from build123d import *

# Parameters (mm, degrees)
F0_W         = 125
F0_H         = 35
F1_DEPTH     = 50
F2_T         = -2.5
F3_T1_DEPTH  = 150
F5_DEPTH     = 47
F6_W         = 123.983182013
F6_H         = 1.5
F7_DEPTH     = 60
F8_T4_DEPTH  = 136.8415969529
F8_T9_DEPTH  = 123.983182013
F8_T14_DEPTH = 136.8415969529


# Not quite as in the source:
# - a fillet or chamfer that OpenCascade refuses, or shapes differently, is made with other operations: its cross-section is extruded or revolved along the edge and cut away or added


with BuildPart() as f1:
    # F0 (on Top) → F1 (new body)
    with BuildSketch(Plane.XY):
        with Locations((-2.4887919426, 0.2054322337)):
            Rectangle(F0_W, F0_H)
    extrude(amount=F1_DEPTH)

    # F2
    f2_openings = [f1.faces().sort_by_distance(p)[0] for p in [
        (-2.488792, 0.205432, 50),
    ]]
    offset(amount=F2_T, openings=f2_openings)

    # F3: fillet of radius 5 on 1 edges, made by hand

    # F3_s2 → F3_t1 (cut)
    with BuildSketch(Plane.YZ.offset(-77.4887919426)):
        with BuildLine():
            ThreePointArc((17.7054322337, 45), (16.2409661396, 48.5355339059), (12.7054322337, 50))
            Line((12.7054322337, 50), (17.7054322337, 50))
            Line((17.7054322337, 50), (17.7054322337, 45))
        make_face()
    extrude(amount=F3_T1_DEPTH, mode=Mode.SUBTRACT)

    # F4 (on Top) → F5 (join)
    with BuildSketch(Plane.XY):
        Polygon((-23.4062603042, 15.2347357944), (-24.9062603042, 15.2233950794), (-24.9062603042, -14.9235967547), (-23.4062603042, -14.9009153247), align=None)
    extrude(amount=F5_DEPTH)

    # F6 (on Top) → F7 (join)
    with BuildSketch(Plane.XY):
        with Locations((-2.1866001189, -18.0445677663)):
            Rectangle(F6_W, F6_H)
    extrude(amount=F7_DEPTH)

    # F8: chamfer of 5 on 1 edges, made by hand


with BuildPart() as f8_tool2:
    # F8_s3 → F8_t4 (new body)
    with BuildSketch(Plane.YZ.offset(-64.1781911254)):
        Polygon((-12.2945677663, 50), (-17.2945677663, 55), (-17.2945677663, 50), align=None)
    extrude(amount=F8_T4_DEPTH)

    split(bisect_by=Plane.YZ.offset(-62.4887919426), keep=Keep.BOTTOM)


with BuildPart() as f1_1:
    add(f1.part)

    # F8_t1: union F8_tool2
    add(f8_tool2.part)


with BuildPart() as f8_tool7:
    # F8_s8 → F8_t9 (new body)
    with BuildSketch(Plane.YZ.offset(-64.1781911254)):
        Polygon((-12.2945677663, 50), (-17.2945677663, 55), (-17.2945677663, 50), align=None)
    extrude(amount=F8_T9_DEPTH)

    split(bisect_by=Plane.XZ.offset(14.7945677663), keep=Keep.TOP)


with BuildPart() as f1_2:
    add(f1_1.part)

    # F8_t6: union F8_tool7
    add(f8_tool7.part)


with BuildPart() as f8_tool12:
    # F8_s13 → F8_t14 (new body)
    with BuildSketch(Plane.YZ.offset(-77.0366060652)):
        Polygon((-12.2945677663, 50), (-17.2945677663, 55), (-17.2945677663, 50), align=None)
    extrude(amount=F8_T14_DEPTH)

    split(bisect_by=Plane.YZ.offset(57.5112080574), keep=Keep.TOP)


with BuildPart() as f1_3:
    add(f1_2.part)

    # F8_t11: union F8_tool12
    add(f8_tool12.part)


solid = f1_3.part
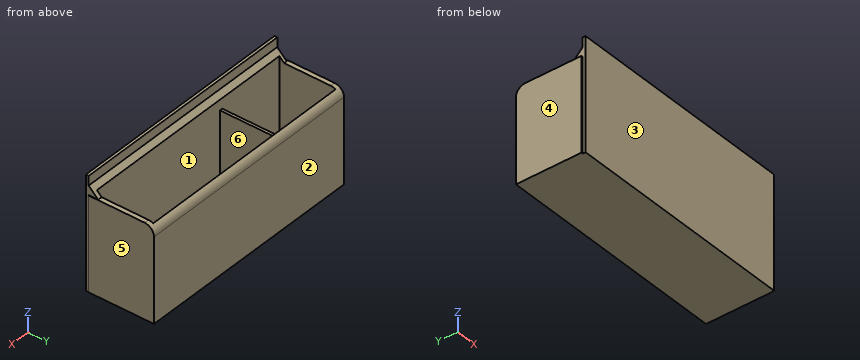
CAD build for the part. Positions are in the model's coordinates, mm. Face numbers are marked on the shaded views. A direction names the side the tool comes from. Coordinates: 2 decimals unless noted, no trailing zeros. Write each loop counter-clockwise with the first axis right and the second up, starting at its lowest first coordinate (ties: lowest second). Pieces come first, ordered by that corner, then holes. Notation, with made-up numbers: (16.5, 0) - (64.5, 0) arc R12 cw to (64.5, 4) - close; hole circle Ø8 at (52.25, 77). An arc over 180 degrees is marked (long way). Use a Markdown table: item, result. Add a question column.
Item 1: Mould opens along Y. For the marked faces 1, 2, 3 and 4 say: pulls with the +Y half, pulls with the -Y half, needs draft (parallel to the pull), parting line crosses it, or undercut.
Item 2: Drill centre lines: L1, parallel to X at y = -0.5, z = 29.5; L2, parallel to Y at x = -13, z = 17; L3, parallel to X at y = -13.5, z = 48.5. Where is each one in solid material? Low to high. Write a range as from..to.
Item 3: Band-saw the part on C-C, the plane y = 11. Give the cut face in (x, z).
Item 4: 3-axis set-ups, long thin cutter, end or side, ignore diameter. For the marked faces 5 and 6: which of +Z, -Z, +X, -X, +Y, -Y reach the whole face in a straight line?
Item 5: Flat gauge pins, fed straight in: pin 1 (12 mm diameter, centred on x = 33.5, y = 6.5, fed in from +Z); pin 2 (3 mm diameter, centred on x = -64, y = -6.5, fed in from +Z); pin 3 (5.5 mm diameter, centred on x = 18.5, z = 57.5, fed in from +Y). Where does each tip first touch, or does it go through?
Item 6: Band-saw the part on B-B, the plane x = 33.5. Give the cut face in (y, z), and give its area (3 significant figures).
Item 7: Band-saw the part on A-A, the plane z = 35. Give the cut face in (x, y) (3 decimals).
Numbers:
| question | item | result |
|---|---|---|
| 1 | face 1 | undercut |
| 1 | face 2 | pulls with the +Y half |
| 1 | face 3 | pulls with the -Y half |
| 1 | face 4 | needs draft |
| 2 | L1 | -64.99..-62.49, -24.91..-23.41, 57.51..60.01 |
| 2 | L2 | -18.79..-14.79, 15.21..17.71 |
| 2 | L3 | -64.99..-62.49, 57.51..60.01 |
| 3 | outline | (-64.99, 0) - (60.01, 0) - (60.01, 50) - (57.51, 50) - (57.51, 2.5) - (-23.41, 2.5) - (-23.41, 47) - (-24.91, 47) - (-24.91, 2.5) - (-62.49, 2.5) - (-62.49, 50) - (-64.99, 50) - close |
| 4 | face 5 | +Z, -Z, +X, +Y, -Y |
| 4 | face 6 | +Z |
| 5 | pin 1 | z = 2.5 |
| 5 | pin 2 | z = 50 |
| 5 | pin 3 | y = -17.04 |
| 6 | outline | (-18.79, 0) - (17.71, 0) - (17.71, 45) arc R5 ccw to (15.21, 49.33) - (15.21, 2.5) - (-14.79, 2.5) - (-14.79, 52.5) - (-17.29, 55) - (-17.29, 60) - (-18.79, 60) - close |
| 6 | area | 420 mm2 |
| 7 | outline | (-64.989, -17.295) - (-64.178, -17.295) - (-64.178, -18.795) - (59.805, -18.795) - (59.805, -17.295) - (60.011, -17.295) - (60.011, 17.705) - (-64.989, 17.705) - close; hole (-62.489, -14.795) - (-24.906, -14.795) - (-24.906, 15.205) - (-62.489, 15.205) - close; hole (-23.406, -14.795) - (57.511, -14.795) - (57.511, 15.205) - (-23.406, 15.205) - close |
